```python
from build123d import *

# Parameters (mm, degrees)
SKETCH1_W           = 25.4
SKETCH1_H           = 25.4
SKETCH1_W_2         = 22.225
SKETCH1_H_2         = 22.225
BOSS_EXTRUDE1_DEPTH = 355.6
SKETCH5_R           = 2.4892
CUT_EXTRUDE2_DEPTH  = 2.54
SKETCH6_R           = 5.715
CUT_EXTRUDE3_DEPTH  = 6.35
SKETCH7_R           = 2.4892
CUT_EXTRUDE4_DEPTH  = 2.54
SKETCH8_R           = 5.75437
CUT_EXTRUDE5_DEPTH  = 2.54
SKETCH10_R          = 2.1828125
CUT_EXTRUDE7_DEPTH  = 25.4


with BuildPart() as part:
    # Sketch1 → Boss-Extrude1 (new body)
    with BuildSketch(Plane.XY):
        Rectangle(SKETCH1_W, SKETCH1_H)
        Rectangle(SKETCH1_W_2, SKETCH1_H_2, mode=Mode.SUBTRACT)
    extrude(amount=BOSS_EXTRUDE1_DEPTH)

    # Sketch5 → Cut-Extrude2 (cut)
    with BuildSketch(Plane.ZY.offset(12.7)):
        with Locations((336.55, 0)):
            Circle(SKETCH5_R)
        with Locations((308.102, 0)):
            Circle(SKETCH5_R)
    extrude(amount=-CUT_EXTRUDE2_DEPTH, mode=Mode.SUBTRACT)

    # Sketch6 → Cut-Extrude3 (cut)
    with BuildSketch(Plane.XZ.offset(12.7)):
        with Locations((0, 228.6)):
            Circle(SKETCH6_R)
        with Locations((0, 153.924)):
            Circle(SKETCH6_R)
    extrude(amount=-CUT_EXTRUDE3_DEPTH, mode=Mode.SUBTRACT)

    # Sketch7 → Cut-Extrude4 (cut)
    with BuildSketch(Plane(origin=(0, 12.7, 0), x_dir=(1, 0, 0), z_dir=(0, 1, 0))):
        with Locations((0, -228.6)):
            Circle(SKETCH7_R)
        with Locations((0, -153.924)):
            Circle(SKETCH7_R)
    extrude(amount=-CUT_EXTRUDE4_DEPTH, mode=Mode.SUBTRACT)

    # Sketch8 → Cut-Extrude5 (cut)
    with BuildSketch(Plane(origin=(12.7, 0, 0), x_dir=(0, 0, -1), z_dir=(1, 0, 0))):
        with Locations((-336.55, 0)):
            Circle(SKETCH8_R)
        with Locations((-308.102, 0)):
            Circle(SKETCH8_R)
    extrude(amount=-CUT_EXTRUDE5_DEPTH, mode=Mode.SUBTRACT)

    # Sketch10 → Cut-Extrude7 (cut)
    with BuildSketch(Plane.ZY.offset(12.7)):
        with Locations((12.7, 0)):
            Circle(SKETCH10_R)
        with Locations((38.1, 0)):
            Circle(SKETCH10_R)
    extrude(amount=-CUT_EXTRUDE7_DEPTH, mode=Mode.SUBTRACT)


solid = part.part
```
Geometry: final body of the model. Coordinates: model frame, mm. A direction names the side the tool comes from. Coordinates: 2 decimals unless noted, no trailing zeros. Order: outer loops, then holes, each group sorted by start corner. A loop starts at its lowest first (then second) coordinate and runs counter-clockwise, first axis right, second up. Notation, with made-up numbers: (49, -4) -> (99, -4) arc R15 ccw to (99, 10) -> close; hole circle Ø2 at (27, 85). An arc over 180 degrees is marked (long way). Write each question's results on one line, items separated by ' | '. Start each with the question number.
1) Set-up query: faces 5 (the cylindrical face through (11.92, 0.25, 313.85)), 6 (the flat face through (0, 11.112, 175)), 7 (the cylindrical face through (-1.24, -11.92, 223.02)), 8 (the flat face through (0, 12.7, 175)). Return all of +Z, -Z, +X, -X, +Y, -Y with unobstructed straight access to the full face (end or side cutting, diameter ignored); none if empty.
2) First-contact query: pin 1 (8 mm diameter, centred on y = 0, z = 308.102, fed in from +X); pin 2 (2 mm diameter, centred on x = 3.5, y = 10, fed in from +Z); pin 3 (6.5 mm diameter, centred on x = 0, z = 228.6, fed in from -Y). Flat tips, straight axial feed; report the tip coordinate or a pass-through.
3) Mould query, pull axis Z, two halves, no side actions, for faces 1 (the flat face through (-12.7, 0, 175)), 2 (the flat face through (-11.3, 0.1, 0)), 3 (the cylindrical face through (11.92, 0.25, 342.3)), 4 (the cylindrical face through (-1.239, -11.917, 148.345)). Classes: released by +Z, released by -Z, zero draft, split by the parting line, or undercut.
4) Cut plane A-A, the plane z = 52. Output: boundary loops of the cut face in (x, y), and give its area (3 significant figures).
5) Material intervals for line 1 along Z through (x, y) = (0, -11.45) (3 decimals); line 2 along X through (y, z) = (-8.25, 176.5), sorted ascending.
Checks:
1) face 5: +X | face 6: +Z, -Z | face 7: -Y | face 8: +Z, -Z, +X, -X, +Y
2) pin 1: x = -11.11 | pin 2: through | pin 3: y = 11.11
3) face 1: zero draft | face 2: released by -Z | face 3: undercut | face 4: undercut
4) outline: (-12.7, -12.7) -> (12.7, -12.7) -> (12.7, 12.7) -> (-12.7, 12.7) -> close; hole (-11.11, -11.11) -> (11.11, -11.11) -> (11.11, 11.11) -> (-11.11, 11.11) -> close | area: 151 mm^2
5) line 1: 0 to 148.209, 159.639 to 222.885, 234.315 to 355.6 | line 2: -12.7 to -11.11, 11.11 to 12.7
